Work out the finished part from the listing and answer in its coordinate system (mm). A direction names the side the tool comes from. Give positions to 0.01 mm unless a question says otherwise; leave off trailing zeros. Order: outer loops, then holes, each group sorted by start corner. A loop starts at its lowest first (then second) coordinate and runs counter-clockwise, first axis right, second up.
```python
from build123d import *

# Parameters (mm, degrees)
SKETCH_1_W                         = 60
SKETCH_1_H                         = 100
SM_BASE_FLANGE_1_DEPTH             = 1.5
SM_EDGE_FLANGE_1_STRIP_W           = 10
SM_EDGE_FLANGE_1_STRIP_H           = 1.5
SM_EDGE_FLANGE_1_STRIP_CUT_DEPTH   = 100
SM_EDGE_FLANGE_1_STRIP_2_W         = 10
SM_EDGE_FLANGE_1_STRIP_2_H         = 1.5
SM_EDGE_FLANGE_1_STRIP_CUT_2_DEPTH = 100
SM_EDGE_FLANGE_1_DEPTH             = 100
SM_EDGE_FLANGE_1_BEND_DEPTH        = 100
SM_EDGE_FLANGE_2_STRIP_W           = 10
SM_EDGE_FLANGE_2_STRIP_H           = 1.5
SM_EDGE_FLANGE_2_STRIP_CUT_DEPTH   = 100
SM_EDGE_FLANGE_2_STRIP_2_W         = 10
SM_EDGE_FLANGE_2_STRIP_2_H         = 1.5
SM_EDGE_FLANGE_2_STRIP_CUT_2_DEPTH = 100
SM_EDGE_FLANGE_2_DEPTH             = 100
SM_EDGE_FLANGE_2_BEND_DEPTH        = 100


# Sheet-metal steps are written as plain solids
with BuildPart() as part:
    # Sketch 1 → 基体-法兰1 (new body)
    with BuildSketch(Plane.XY):
        Rectangle(SKETCH_1_W, SKETCH_1_H)
    extrude(amount=-SM_BASE_FLANGE_1_DEPTH)

    # 边线-法兰1 strip (across the edge) → 边线-法兰1 strip cut (cut)
    with BuildSketch(Plane(origin=(-30, 50, 0), x_dir=(1, 0, 0), z_dir=(0, -1, 0))):
        with Locations((-1.5, -0.75)):
            Rectangle(SM_EDGE_FLANGE_1_STRIP_W, SM_EDGE_FLANGE_1_STRIP_H)
    extrude(amount=SM_EDGE_FLANGE_1_STRIP_CUT_DEPTH, mode=Mode.SUBTRACT)

    # 边线-法兰1 strip 2 (across the edge) → 边线-法兰1 strip cut 2 (cut)
    with BuildSketch(Plane(origin=(30, -50, 0), x_dir=(-1, 0, 0), z_dir=(0, 1, 0))):
        with Locations((-1.5, -0.75)):
            Rectangle(SM_EDGE_FLANGE_1_STRIP_2_W, SM_EDGE_FLANGE_1_STRIP_2_H)
    extrude(amount=SM_EDGE_FLANGE_1_STRIP_CUT_2_DEPTH, mode=Mode.SUBTRACT)

    # 边线-法兰1 section (across the edge) → 边线-法兰1 (add)
    with BuildSketch(Plane(origin=(-30, 50, 0), x_dir=(1, 0, 0), z_dir=(0, -1, 0))):
        with BuildLine():
            Line((0, 2), (0, 13.5))
            Line((0, 13.5), (1.5, 13.5))
            Line((1.5, 13.5), (1.5, 2))
            ThreePointArc((1.5, 2), (2.085786438, 0.585786438), (3.5, 0))
            Line((3.5, 0), (3.5, -1.5))
            ThreePointArc((3.5, -1.5), (1.025126266, -0.474873734), (0, 2))
        make_face()
    extrude(amount=SM_EDGE_FLANGE_1_DEPTH)

    # 边线-法兰1 section 2 (across the edge) → 边线-法兰1 bend (add)
    with BuildSketch(Plane(origin=(30, -50, 0), x_dir=(-1, 0, 0), z_dir=(0, 1, 0))):
        with BuildLine():
            Line((0, 2), (0, 13.5))
            Line((0, 13.5), (1.5, 13.5))
            Line((1.5, 13.5), (1.5, 2))
            ThreePointArc((1.5, 2), (2.085786438, 0.585786438), (3.5, 0))
            Line((3.5, 0), (3.5, -1.5))
            ThreePointArc((3.5, -1.5), (1.025126266, -0.474873734), (0, 2))
        make_face()
    extrude(amount=SM_EDGE_FLANGE_1_BEND_DEPTH)

    # 边线-法兰2 strip (across the edge) → 边线-法兰2 strip cut (cut)
    with BuildSketch(Plane(origin=(-30, -50, 13.5), x_dir=(0, 0, -1), z_dir=(0, 1, 0))):
        with Locations((-1.5, -0.75)):
            Rectangle(SM_EDGE_FLANGE_2_STRIP_W, SM_EDGE_FLANGE_2_STRIP_H)
    extrude(amount=SM_EDGE_FLANGE_2_STRIP_CUT_DEPTH, mode=Mode.SUBTRACT)

    # 边线-法兰2 strip 2 (across the edge) → 边线-法兰2 strip cut 2 (cut)
    with BuildSketch(Plane(origin=(30, 50, 13.5), x_dir=(0, 0, -1), z_dir=(0, -1, 0))):
        with Locations((-1.5, -0.75)):
            Rectangle(SM_EDGE_FLANGE_2_STRIP_2_W, SM_EDGE_FLANGE_2_STRIP_2_H)
    extrude(amount=SM_EDGE_FLANGE_2_STRIP_CUT_2_DEPTH, mode=Mode.SUBTRACT)

    # 边线-法兰2 section (across the edge) → 边线-法兰2 (add)
    with BuildSketch(Plane(origin=(-30, -50, 13.5), x_dir=(0, 0, -1), z_dir=(0, 1, 0))):
        with BuildLine():
            Line((0, 2), (0, 13.5))
            Line((0, 13.5), (1.5, 13.5))
            Line((1.5, 13.5), (1.5, 2))
            ThreePointArc((1.5, 2), (2.085786438, 0.585786438), (3.5, 0))
            Line((3.5, 0), (3.5, -1.5))
            ThreePointArc((3.5, -1.5), (1.025126266, -0.474873734), (0, 2))
        make_face()
    extrude(amount=SM_EDGE_FLANGE_2_DEPTH)

    # 边线-法兰2 section 2 (across the edge) → 边线-法兰2 bend (add)
    with BuildSketch(Plane(origin=(30, 50, 13.5), x_dir=(0, 0, -1), z_dir=(0, -1, 0))):
        with BuildLine():
            Line((0, 2), (0, 13.5))
            Line((0, 13.5), (1.5, 13.5))
            Line((1.5, 13.5), (1.5, 2))
            ThreePointArc((1.5, 2), (2.085786438, 0.585786438), (3.5, 0))
            Line((3.5, 0), (3.5, -1.5))
            ThreePointArc((3.5, -1.5), (1.025126266, -0.474873734), (0, 2))
        make_face()
    extrude(amount=SM_EDGE_FLANGE_2_BEND_DEPTH)


solid = part.part
```
1. The mould has two halves that part along X. Classify faces 6 (the face through (29.5, 0.7, 12.45)), 7 (the face through (3, -50, -1)), 8 (the face through (30, -1, 6)): pulls with the +X half, pulls with the -X half, needs draft (parallel to the pull), parting line crosses it, or undercut.
Findings below:
face 6: undercut
face 7: needs draft
face 8: pulls with the +X half
2. The part is cut by section A-A (z = 3.5). Write down the section's boundary in (x, y), then the cut area to 3 significant figures.
Findings below:
outline: (-30, -50) - (-28.5, -50) - (-28.5, 50) - (-30, 50) - close; (28.5, -50) - (30, -50) - (30, 50) - (28.5, 50) - close
area: 300 mm2
3. The part is cut by section C-C (x = -20). Write down the section's boundary in (y, z), then the cut area to 3 significant figures.
Findings below:
outline: (-50, -1.5) - (50, -1.5) - (50, 0) - (-50, 0) - close
area: 150 mm2
4. The part is cut by section B-B (y = -4.5). Write down the section's boundary in (x, z).
Findings below:
outline: (-43.5, 12) - (-32, 12) arc R2 cw to (-30, 10) - (-30, 2) arc R3.5 ccw to (-26.5, -1.5) - (26.5, -1.5) arc R3.5 ccw to (30, 2) - (30, 10) arc R2 cw to (32, 12) - (43.5, 12) - (43.5, 13.5) - (32, 13.5) arc R3.5 ccw to (28.5, 10) - (28.5, 2) arc R2 cw to (26.5, 0) - (-26.5, 0) arc R2 cw to (-28.5, 2) - (-28.5, 10) arc R3.5 ccw to (-32, 13.5) - (-43.5, 13.5) - close
5. Given P1, Ø4, axis at x = 21.5, y = -10.5, coming from the +Z side; P2, Ø6, axis at x = 39, y = -21, coming from the -Z side; P3, Ø6.5, axis at y = -12.5, z = 5, coming from the -X side; P4, Ø1, axis at x = 16.5, z = 1.5, coming from the +Y side, each flat-ended and moving along its own axis, determine where each tip first touches the part or whether it passes through.
Findings below:
P1: stops at z = 0
P2: stops at z = 12
P3: stops at x = -30
P4: passes through
6. Which of the six approach directions +Z, -Z, +X, -X, +Y, -Y give full straight-line access (tool end or side, diameter ignored) to faces 1 (the face through (38, 1, 13.5)), 2 (the face through (-38, -1, 12)), 3 (the face through (3, 50, -1)), 4 (the face through (38, 1, 12)), 5 (the face through (28.5, -1, 6))?
Findings below:
face 1: +Z, +X, -X, +Y, -Y
face 2: -Z, -X, +Y, -Y
face 3: +Z, -Z, +X, -X, +Y
face 4: -Z, +X, +Y, -Y
face 5: +Z, +Y, -Y
7. Straight lines are drawn through the part: probe 1 along X at (y, z) = (-20.5, 8.5); probe 2 along Z at (x, y) = (12, 35.5); probe 3 along X at (y, z) = (-1.5, 0.5). For each, find the intervals that lie inside material, in ascending order.
Findings below:
probe 1: x = -30 to -28.5, 28.5 to 30
probe 2: z = -1.5 to 0
probe 3: x = -29.66 to -27.82, 27.82 to 29.66
